from build123d import *

# Parameters (mm, degrees)
SKETCH2_R           = 4.066
BOSS_EXTRUDE1_DEPTH = 15.875
SKETCH3_R           = 9.525
BOSS_EXTRUDE2_DEPTH = 8.255
CUT_EXTRUDE1_DEPTH  = 3.875


with BuildPart() as part:
    # Sketch2 → Boss-Extrude1 (new body)
    with BuildSketch(Plane(origin=(0, 0, 0), x_dir=(1, 0, 0), z_dir=(0, 1, 0))):
        with Locations(Location((0, 0, 0), (0, 0, 270))):
            Circle(SKETCH2_R)
    extrude(amount=BOSS_EXTRUDE1_DEPTH)

    # Sketch3 → Boss-Extrude2 (add)
    with BuildSketch(Plane(origin=(0, 15.875, 0), x_dir=(1, 0, 0), z_dir=(0, 1, 0))):
        with Locations(Location((0, 0, 0), (0, 0, 270))):
            Circle(SKETCH3_R)
    extrude(amount=BOSS_EXTRUDE2_DEPTH)

    # Sketch4 → Cut-Extrude1 (cut)
    with BuildSketch(Plane(origin=(0, 24.13, 0), x_dir=(1, 0, 0), z_dir=(0, 1, 0))):
        with BuildLine():
            Line((-2.439590334, 2.032), (2.439590334, 2.032))
            ThreePointArc((2.439590334, 2.032), (0, -3.175), (-2.439590334, 2.032))
        make_face()
    extrude(amount=-CUT_EXTRUDE1_DEPTH, mode=Mode.SUBTRACT)


solid = part.part
Source: CAD feature listing. Evaluate the final solid. Frame: model axes, mm. A direction names the side the tool comes from. Round coordinates to 2 decimals unless told otherwise and drop trailing zeros. Loops run counter-clockwise (first coordinate to the right, second up) from the corner with the lowest first, then second, coordinate; pieces in that order, holes last. Notation, with made-up numbers: (-14, 22) - (42, 22) arc R29 ccw to (42, 56) - close; hole circle Ø2 at (55, -14). An arc over 180 degrees is marked (long way). Write item = value, one per line. Start each with the question number.
(1) Set-up query: faces 4 (the face through (0.1, 24.13, -2.3)), 5 (the face through (0, 22, -2.032)), 6 (the face through (-4, 15.875, 2)). Return all of +Z, -Z, +X, -X, +Y, -Y with unobstructed straight access to the full face (end or side cutting, diameter ignored); none if empty.
(2) Section query C-C, the plane y = 19.25. Output: boundary loops of the cut face in (x, z) (3 decimals), plus the area to 3 significant figures.
(3) Pull-direction query (X, two-part tool) for faces 1 (the face through (0, 0, 0)), 2 (the face through (0, 20.255, 1)), 3 (the face through (-5.796, 19.945, -7.559)); classes: +X half, -X half, draft (parallel to the pull), parting line (faces both ways), or undercut.
(4) Section query B-B, the plane x = 0. Output: boundary loops of the cut face in (y, z) (3 decimals), plus the area to 3 significant figures.
(5) Section query D-D, the plane x = -3.5. Output: boundary loops of the cut face in (y, z) (3 decimals), plus the area to 3 significant figures.
(6) Ray query, line 1 along X through (y, z) = (22.2, 0) (3 decimals); line 2 along Y through (x, z) = (2.75, 1) (3 decimals); line 3 along Y through (x, z) = (5, -1.5) (3 decimals). Return the intervals inside material, ascending. Write a range as from..to.
(7) Section query A-A, the plane z = 0. Output: boundary loops of the cut face in (x, y) (3 decimals), plus the area to 3 significant figures.
(8) Pin query (flat end, axial travel): pin 1 (4 mm diameter, centred on y = 12, z = 1.5, fed in from +X); pin 2 (1.5 mm diameter, centred on y = 3.5, z = -2.5, fed in from -X); pin 3 (1.2 mm diameter, centred on x = -1, y = 23, fed in from +Z). Return the tip coordinate at first contact, or that it passes through.
Conclusion:
q1.face_4 = +Z, -Z, +X, -X, +Y
q1.face_5 = +Y
q1.face_6 = -Y
q2.outline = circle Ø19.05 at (0, 0)
q2.area = 285 mm2
q3.face_1 = draft
q3.face_2 = undercut
q3.face_3 = parting line
q4.outline = (0, -4.066) - (15.875, -4.066) - (15.875, -9.525) - (24.13, -9.525) - (24.13, -2.032) - (20.255, -2.032) - (20.255, 3.175) - (24.13, 3.175) - (24.13, 9.525) - (15.875, 9.525) - (15.875, 4.066) - (0, 4.066) - close
q4.area = 266 mm2
q5.outline = (0, -2.069) - (15.875, -2.069) - (15.875, -8.859) - (24.13, -8.859) - (24.13, 8.859) - (15.875, 8.859) - (15.875, 2.069) - (0, 2.069) - close
q5.area = 212 mm2
q6.line_1 = -9.525..-3.175, 3.175..9.525
q6.line_2 = 0..20.255
q6.line_3 = 15.875..24.13
q7.outline = (-9.525, 15.875) - (-4.066, 15.875) - (-4.066, 0) - (4.066, 0) - (4.066, 15.875) - (9.525, 15.875) - (9.525, 24.13) - (3.175, 24.13) - (3.175, 20.255) - (-3.175, 20.255) - (-3.175, 24.13) - (-9.525, 24.13) - close
q7.area = 262 mm2
q8.pin_1 = 4.07
q8.pin_2 = -3.67
q8.pin_3 = 9.52
